The listing builds one solid part. Answer for the finished solid, in the listing's coordinates (mm). Face numbers are marked on the shaded views. A direction names the side the tool comes from. Coordinates: 2 decimals unless noted, no trailing zeros. Loops run counter-clockwise (first coordinate to the right, second up) from the corner with the lowest first, then second, coordinate; pieces in that order, holes last. Notation, with made-up numbers: (18.25, -7) - (51.25, -7) arc R13 cw to (51.25, 16) - close; hole circle Ø7 at (-24, 52). An arc over 180 degrees is marked (long way). Return JSON: item names as keys, results as strings. Group by question number.
1. Section A-A (y = 12.5) is taken. Write down the section's boundary in (x, z).
2. Which of the six approach directions +Z, -Z, +X, -X, +Y, -Y give full straight-line access (tool end or side, diameter ignored) to the marked faces 1 and 2?
3. Section D-D (z = 15.75) is taken. Write down the section's boundary in (x, y).
4. Section C-C (x = 34) is taken. Write down the section's boundary in (y, z).
5. Find the intervals of material crossed by line 1 along X through (y, z) = (12.5, 1.05); line 2 along Z through (x, y) = (66, 14); line 3 along Y through (x, z) = (112.5, 1.45), in increasing order.
6. Each of these flat-tipped pins is pushed along its axis until it touches: P1, Ø5, axis at x = 40, y = -9.5, coming from the +Z side; P2, Ø3.5, axis at x = 112.5, y = 12.5, coming from the -Z side (3 decimals); P3, Ø8, axis at x = 31, y = -10.5, coming from the +Z side; P4, Ø8, axis at x = 67, z = 16, coming from the +Y side. Where does it stop, or does it pass through?
7. Section B-B (x = 12.5) is taken. Write down the section's boundary in (y, z).
```python
from build123d import *

# Parameters (mm, degrees)
F1_DEPTH = 125
F2_R     = 2.3114
F3_DEPTH = 25
F4_R     = 2.3114
F5_DEPTH = 25


with BuildPart() as f1:
    # F0 (on Right) → F1 (new body)
    with BuildSketch(Plane.YZ):
        Polygon((-17.67767, 17.67767), (0, 0), (25, 0), (25, 3), (1.242641, 3), (-15.556349, 19.79899), align=None)
    extrude(amount=F1_DEPTH)

    # F2 (on face) → F3 (cut)
    with BuildSketch(Plane(origin=(0, 0, 0), x_dir=(1, 0, 0), z_dir=(0, 0, -1))):
        with Locations((12.5, -12.5)):
            Circle(F2_R)
        with Locations((112.5, -12.5)):
            Circle(F2_R)
    extrude(amount=-F3_DEPTH, mode=Mode.SUBTRACT)

    # F4 (on face) → F5 (cut)
    with BuildSketch(Plane(origin=(0, 0, 0), x_dir=(1, 0, 0), z_dir=(0, -0.707107, -0.707107))):
        with Locations((12.5, 12.5)):
            Circle(F4_R)
        with Locations((112.5, 12.5)):
            Circle(F4_R)
    extrude(amount=-F5_DEPTH, mode=Mode.SUBTRACT)


solid = f1.part
```
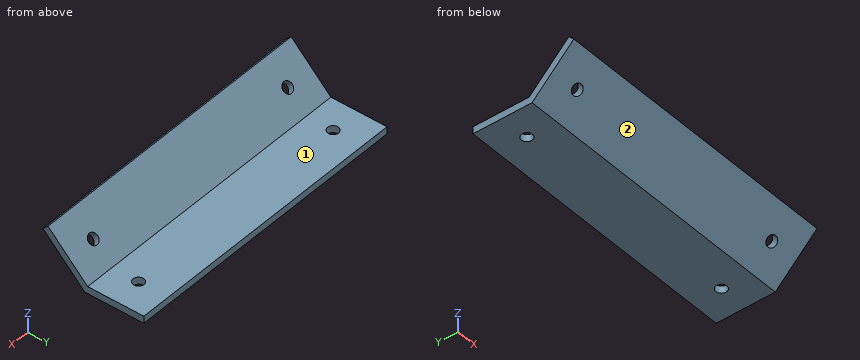
The answers:
{
 "1": {"outline": "(0, 0) - (10.19, 0) - (10.19, 3) - (0, 3) - close; (14.81, 0) - (110.19, 0) - (110.19, 3) - (14.81, 3) - close; (114.81, 0) - (125, 0) - (125, 3) - (114.81, 3) - close"},
 "2": {"face 1": "+Z, +X, -X, +Y", "face 2": "-Z, +X, -X, -Y"},
 "3": {"outline": "(0, -15.75) - (125, -15.75) - (125, -11.51) - (0, -11.51) - close"},
 "4": {"outline": "(-17.68, 17.68) - (0, 0) - (25, 0) - (25, 3) - (1.24, 3) - (-15.56, 19.8) - close"},
 "5": {"line 1": "x = 0 to 10.19, 14.81 to 110.19, 114.81 to 125", "line 2": "z = 0 to 3", "line 3": "y = -1.45 to 10.19, 14.81 to 25"},
 "6": {"P1": "stops at z = 16.24", "P2": "passes through", "P3": "stops at z = 18.74", "P4": "stops at y = -7.76"},
 "7": {"outline": "(-17.68, 17.68) - (-10.47, 10.47) - (-8.35, 12.59) - (-15.56, 19.8) - close; (-7.2, 7.2) - (0, 0) - (10.19, 0) - (10.19, 3) - (1.24, 3) - (-5.08, 9.33) - close; (14.81, 0) - (25, 0) - (25, 3) - (14.81, 3) - close"}
}
